For this review, take the finished solid that the model builds, in its own axes (mm). A direction names the side the tool comes from. Coordinates: 2 decimals unless noted, no trailing zeros. Write each loop counter-clockwise with the first axis right and the second up, starting at its lowest first coordinate (ties: lowest second). Pieces come first, ordered by that corner, then holes. Notation, with made-up numbers: (33, 61.5) -> (49, 61.5) arc R13 cw to (49, 72.5) -> close; hole circle Ø7 at (30.5, 77). An arc over 180 degrees is marked (long way). One line per item, written item: value. Start each with the question number.
1) Add section B-B (x = -28.5). State the section outline as (y, z) points, and give its area (3 significant figures).
2) Add section C-C (z = 15.5). State the section outline as (x, y) points.
3) For pin 1 Ø2 at (y, z) = (-72.05, 27.13) entering from -X; pin 2 Ø2 at (x, z) = (-52, 38.5) entering from -Y, all flat-tipped, find the tip position at first contact; note any pin that passes through.
4) Mouldability with a two-part tool opening along Y and no side actions: class faces 3 (the cylindrical face through (-74.757, -73.184, 27.485)), 4 (the flat face through (-39, -38, 0)), 5 (the flat face through (-39, 0, 26)), 6 (the cylindrical face through (-1.28, -74.34, 29.49)) as released by +Y, released by -Y, zero draft, split by the parting line, or undercut.
5) Machinability: for faces 1 (the flat face through (-39, -38, 50.8)), 2 (the flat face through (-73.274, -40, 25)), which of the approach directions +Z, -Z, +X, -X, +Y, -Y give a long, thin tool a straight path to every point of the face, cutting with its end or side? Answer none if there is none.
6) For probe 1 along X at (y, z) = (-63, 25); probe 2 along Z at (x, y) = (-42, -20.5); probe 3 along Y at (x, z) = (-67.5, 21), list the stretches that pass through material, from the lowest coordinate up. Write a range as from..to.
7) Add section A-A (y = -5.5). State the section outline as (x, z) points, and give its area (3 significant figures).
from build123d import *

# Parameters (mm, degrees)
F0_W     = 76.2
F0_H     = 50.8
F1_DEPTH = 76.2
F2_W     = 70.673531
F2_H     = 45.6187
F3_DEPTH = 73.66
F4_R     = 1.188215
F5_DEPTH = 5.08
F6_R     = 1.1938
F7_DEPTH = 5.08


with BuildPart() as f1:
    # F0 (on Front) → F1 (new body)
    with BuildSketch(Plane.XZ):
        with Locations((-38.1, 25.4)):
            Rectangle(F0_W, F0_H)
    extrude(amount=F1_DEPTH)

    # F2 (on face) → F3 (cut)
    with BuildSketch(Plane.XZ.offset(76.2)):
        with Locations((-37.936796, 25.291196)):
            Rectangle(F2_W, F2_H)
    extrude(amount=-F3_DEPTH, mode=Mode.SUBTRACT)

    # F4 (on face) → F5 (cut)
    with BuildSketch(Plane(origin=(-76.2, 0, 0), x_dir=(0, -1, 0), z_dir=(-1, 0, 0))):
        with Locations((72.051063, 27.127683)):
            Circle(F4_R)
    extrude(amount=-F5_DEPTH, mode=Mode.SUBTRACT)

    # F6 (on face) → F7 (cut)
    with BuildSketch(Plane.YZ):
        with Locations((-73.146977, 29.433548)):
            Circle(F6_R)
    extrude(amount=-F7_DEPTH, mode=Mode.SUBTRACT)


solid = f1.part
Numbers:
1. outline: (-76.2, 0) -> (0, 0) -> (0, 50.8) -> (-76.2, 50.8) -> (-76.2, 48.1) -> (-2.54, 48.1) -> (-2.54, 2.48) -> (-76.2, 2.48) -> close
1. area: 511 mm²
2. outline: (-76.2, -76.2) -> (-73.27, -76.2) -> (-73.27, -2.54) -> (-2.6, -2.54) -> (-2.6, -76.2) -> (0, -76.2) -> (0, 0) -> (-76.2, 0) -> close
3. pin 1: x = -2.6
3. pin 2: y = -2.54
4. face 3: undercut
4. face 4: zero draft
4. face 5: released by +Y
4. face 6: undercut
5. face 1: +Z, +X, -X, +Y, -Y
5. face 2: -Y
6. probe 1: -76.2..-73.27, -2.6..0
6. probe 2: 0..2.48, 48.1..50.8
6. probe 3: -2.54..0
7. outline: (-76.2, 0) -> (0, 0) -> (0, 50.8) -> (-76.2, 50.8) -> close; hole (-73.27, 2.48) -> (-2.6, 2.48) -> (-2.6, 48.1) -> (-73.27, 48.1) -> close
7. area: 647 mm²
